```python
from build123d import *

# Parameters (mm, degrees)
SKETCH1_W          = 70
SKETCH1_H          = 10
EXTRUDE1_DEPTH     = 58
SKETCH2_R          = 5
EXTRUDE2_DEPTH     = 26
CUT_EXTRUDE1_DEPTH = 30
CHAMFER1_SIZE      = 15
FILLET1_R          = 3
SKETCH4_R          = 1.8
CUT_EXTRUDE2_DEPTH = 60


with BuildPart() as part:
    # Sketch1 → Extrude1 (new body)
    with BuildSketch(Plane.XY.offset(-7.106345979)):
        with Locations((-10.032216865, -100)):
            Rectangle(SKETCH1_W, SKETCH1_H)
    extrude(amount=EXTRUDE1_DEPTH)

    # Sketch2 → Extrude2 (add)
    with BuildSketch(Plane.XZ.offset(105)):
        with Locations(Location((-35.032216865, 21.593654021, 0), (0, 0, 180))):
            Circle(SKETCH2_R)
    extrude(amount=EXTRUDE2_DEPTH)

    # Sketch3 → Cut-Extrude1 (cut)
    with BuildSketch(Plane.XZ.offset(105)):
        with BuildLine():
            Line((-20.032216865, 42.893654021), (11.967783135, 42.893654021))
            ThreePointArc((11.967783135, 42.893654021), (15.503317041, 41.429187927), (16.967783135, 37.893654021))
            Line((16.967783135, 37.893654021), (16.967783135, 5.893654021))
            ThreePointArc((16.967783135, 5.893654021), (15.503317041, 2.358120115), (11.967783135, 0.893654021))
            Line((11.967783135, 0.893654021), (-20.032216865, 0.893654021))
            ThreePointArc((-20.032216865, 0.893654021), (-23.567750771, 2.358120115), (-25.032216865, 5.893654021))
            Line((-25.032216865, 5.893654021), (-25.032216865, 37.893654021))
            ThreePointArc((-25.032216865, 37.893654021), (-23.567750771, 41.429187927), (-20.032216865, 42.893654021))
        make_face()
    extrude(amount=-CUT_EXTRUDE1_DEPTH, mode=Mode.SUBTRACT)

    # Chamfer1
    chamfer1_edges = [part.edges().sort_by_distance(p)[0] for p in [
        (-45.032216865, -100, 50.893654021),
        (-45.032216865, -100, -7.106345979),
    ]]
    chamfer(chamfer1_edges, length=CHAMFER1_SIZE)

    # Fillet1
    fillet1_edges = [part.edges().sort_by_distance(p)[0] for p in [
        (-45.032216865, -100, 35.893654021),
        (-45.032216865, -100, 7.893654021),
    ]]
    fillet(fillet1_edges, radius=FILLET1_R)

    # Sketch4 → Cut-Extrude2 (cut)
    with BuildSketch(Plane.XY.offset(50.893654021)):
        with Locations((-20.032216865, -100)):
            Circle(SKETCH4_R)
        with Locations((-0.032216865, -100)):
            Circle(SKETCH4_R)
        with Locations((19.967783135, -100)):
            Circle(SKETCH4_R)
    extrude(amount=-CUT_EXTRUDE2_DEPTH, mode=Mode.SUBTRACT)


solid = part.part
```
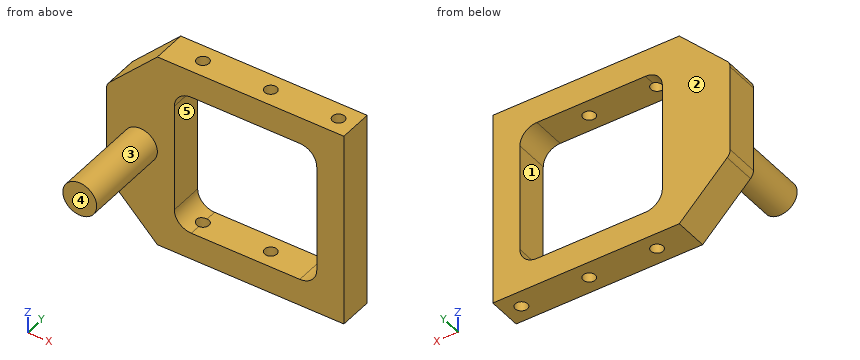
Geometry check sheet. Reference: the model listing, model coordinates, mm. Face numbers are marked on the shaded views. A direction names the side the tool comes from. Give positions to 0.01 mm unless a question says otherwise; leave off trailing zeros. Write each loop counter-clockwise with the first axis right and the second up, starting at its lowest first coordinate (ties: lowest second). Pieces come first, ordered by that corner, then holes. Notation, with made-up numbers: (38.5, 17.5) -> (79.5, 17.5) arc R17 cw to (79.5, 22.5) -> close; hole circle Ø5 at (23, -8). An arc over 180 degrees is marked (long way). One line per question, with ' | ' between items.
Item 1: Sectioned sample at D-D, the plane z = 4. Record the boundary of the cut face in (x, y), plus the area to 3 significant figures.
Determined:
outline: (-41.14, -105) -> (-24.66, -105) -> (-24.66, -95) -> (-41.14, -95) -> close; (16.6, -105) -> (24.97, -105) -> (24.97, -95) -> (16.6, -95) -> close; hole circle Ø3.6 at (19.97, -100) | area: 238 mm^2
Item 2: Depth check by flat-ended pin: pin 1 (17.5 mm diameter, centred on x = -24, z = 13, fed in from -Y). Enter the tip coordinate at first touch or a pass-through.
Determined:
pin 1: y = -105
Item 3: Sectioned sample at B-B, the plane z = 30.5. Record the boundary of the cut face in (x, y).
Determined:
outline: (-45.03, -105) -> (-25.03, -105) -> (-25.03, -95) -> (-45.03, -95) -> close; (16.97, -105) -> (24.97, -105) -> (24.97, -95) -> (16.97, -95) -> close; hole circle Ø3.6 at (19.97, -100)
Item 4: Draft check along X on the marked faces 1, 2 and 3. Enter one of: released by +X, released by -X, zero draft, split by the parting line, or undercut.
Determined:
face 1: undercut | face 2: zero draft | face 3: split by the parting line
Item 5: Scan lines: line 1 along X through (y, z) = (-100, 46); line 2 along X through (y, z) = (-104, 31); line 3 along X through (y, z) = (-100, -1). Record each from-to range of solid material in increasing order.
Determined:
line 1: -34.93 to -21.83, -18.23 to -1.83, 1.77 to 18.17, 21.77 to 24.97 | line 2: -45.03 to -25.03, 16.97 to 24.97 | line 3: -36.14 to -21.83, -18.23 to -1.83, 1.77 to 18.17, 21.77 to 24.97
Item 6: Access from +Z, -Z, +X, -X, +Y, -Y to the whole of each face (thin tool, end or side, straight path). Record for the marked faces 4 and 5.
Determined:
face 4: +Z, -Z, +X, -X, -Y | face 5: +Y, -Y
Item 7: Sectioned sample at A-A, the plane x = -15. Record the boundary of the cut face in (y, z), plus the area to 3 significant figures.
Determined:
outline: (-105, -7.11) -> (-95, -7.11) -> (-95, 0.89) -> (-105, 0.89) -> close; (-105, 42.89) -> (-95, 42.89) -> (-95, 50.89) -> (-105, 50.89) -> close | area: 160 mm^2
Item 8: Sectioned sample at C-C, the plane y = -100. State how many separate pieces and enclosed holes the cut face has, plus the area to 3 significant figures.
Determined:
separate pieces: 5 | enclosed holes: 0 | area: 1,770 mm^2
